from build123d import *

# Parameters (mm, degrees)
F0_W     = 500
F0_H     = 500
F1_DEPTH = 50.8
F3_D     = 5.1054
F4_SIZE  = 50.8


with BuildPart() as f1:
    # F0 (on Top) → F1 (new body)
    with BuildSketch(Plane.XY):
        Rectangle(F0_W, F0_H)
    extrude(amount=F1_DEPTH)

    # F3 (through all)
    with Locations(Plane.XY.offset(50.8)):
        with Locations((-85.9357491136, 151.999682188)):
            Hole(F3_D / 2)

    # F4
    f4_edges = [f1.edges().sort_by_distance(p)[0] for p in [
        (-250, 250, 25.4),
        (-250, -250, 25.4),
        (250, -250, 25.4),
        (250, 250, 25.4),
    ]]
    chamfer(f4_edges, length=F4_SIZE)


solid = f1.part
Check sheet for the modelled part. Datum: model origin and axes. Units: mm. Round coordinates to 2 decimals unless told otherwise and drop trailing zeros. Loops run counter-clockwise (first coordinate to the right, second up) from the corner with the lowest first, then second, coordinate; pieces in that order, holes last. Notation, with made-up numbers: M 17.5,65 L 54.5,65 A9 ccw 54.5,75 Z; hole C -24.5,50.25 d5. An arc over 180 degrees is marked long. One line per item, written item: value.
(1) Sectioned sample at B-B, the plane y = 212. Record the cut outline in (x, z), then the cut area to 3 significant figures.
Computed values:
outline: M -237.2,0 L 237.2,0 L 237.2,50.8 L -237.2,50.8 Z
area: 24,100 mm^2
(2) Sectioned sample at A-A, the plane z = 6.5. Record the cut outline in (x, y), then the cut area to 3 significant figures.
Computed values:
outline: M -250,-199.2 L -199.2,-250 L 199.2,-250 L 250,-199.2 L 250,199.2 L 199.2,250 L -199.2,250 L -250,199.2 Z; hole C -85.94,152 d5.11
area: 245,000 mm^2
(3) Thickness scan on line 1 (Y direction, x = 217, z = 43.5); line 2 (X direction, y = 210, z = 16.5). Record the ranges inside material, lowest first.
Computed values:
line 1: y = -232.2 to 232.2
line 2: x = -239.2 to 239.2
